from build123d import *

# Parameters (mm, degrees)
PAD_DEPTH    = 4
PAD001_DEPTH = 3
POCKET_DEPTH = 7.001


with BuildPart() as part:
    # Sketch → Pad (new body)
    with BuildSketch(Plane.XY):
        with BuildLine():
            ThreePointArc((0, 3.5), (-3.5, 0), (0, -3.5))
            Line((0, -3.5), (10, -3.5))
            ThreePointArc((10, -3.5), (13.5, 0), (10, 3.5))
            Line((0, 3.5), (10, 3.5))
        make_face()
    extrude(amount=PAD_DEPTH)

    # Sketch001 (on Face6 of Pad) → Pad001 (join)
    with BuildSketch(Plane.XY.offset(4)):
        with BuildLine():
            ThreePointArc((0, 1.85), (-1.85, 0), (0, -1.85))
            Line((0, -1.85), (10, -1.85))
            ThreePointArc((10, -1.85), (11.85, 0), (10, 1.85))
            Line((0, 1.85), (10, 1.85))
        make_face()
    extrude(amount=PAD001_DEPTH)

    # Sketch002 (on Face11 of Pad001) → Pocket (cut, through all)
    with BuildSketch(Plane.XY.offset(7)):
        with BuildLine():
            ThreePointArc((8.35, 0), (6.6, 1.75), (4.85, 0))
            Line((4.85, -3.5), (4.85, 0))
            Line((8.35, -3.5), (4.85, -3.5))
            Line((8.35, 0), (8.35, -3.5))
        make_face()
    extrude(amount=-POCKET_DEPTH, mode=Mode.SUBTRACT)


solid = part.part
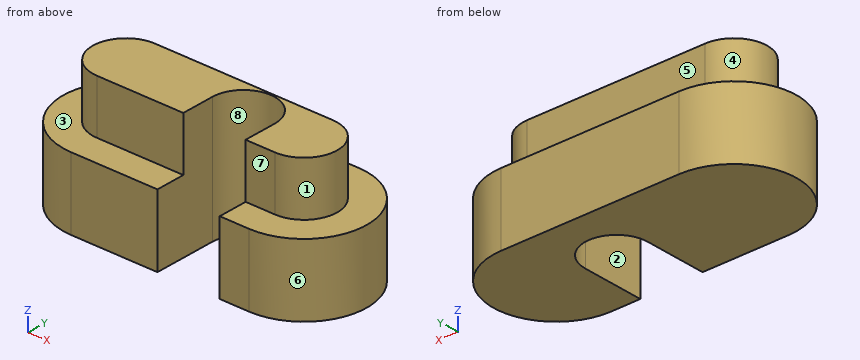
Check sheet for the modelled part. Datum: model origin and axes. Units: mm. Face numbers are marked on the shaded views. A direction names the side the tool comes from. Round coordinates to 2 decimals unless told otherwise and drop trailing zeros. Loops run counter-clockwise (first coordinate to the right, second up) from the corner with the lowest first, then second, coordinate; pieces in that order, holes last. Notation, with made-up numbers: M 30,49.5 L 63,49.5 A9 ccw 63,58.5 Z; hole C -17,37 d1. An arc over 180 degrees is marked long. One line per item, written item: value.
(1) Sectioned sample at A-A, the plane y = -1. Record the cut outline in (x, z), then the cut area to 3 significant figures.
Computed values:
outline: M -3.35,0 L 4.85,0 L 4.85,7 L -1.56,7 L -1.56,4 L -3.35,4 Z; M 8.35,0 L 13.35,0 L 13.35,4 L 11.56,4 L 11.56,7 L 8.35,7 Z
area: 81.7 mm^2
(2) Sectioned sample at D-D, the plane y = -0.25. Record the cut outline in (x, z).
Computed values:
outline: M -3.49,0 L 4.85,0 L 4.85,7 L -1.83,7 L -1.83,4 L -3.49,4 Z; M 8.35,0 L 13.49,0 L 13.49,4 L 11.83,4 L 11.83,7 L 8.35,7 Z
(3) Thickness scan on line 1 (X direction, y = 1.5, z = 5.75); line 2 (X direction, y = -2.75, z = 3.5); line 3 (Z direction, x = 0.25, y = 2.75). Record the ranges inside material, lowest first.
Computed values:
line 1: x = -1.08 to 5.7, 7.5 to 11.08
line 2: x = -2.17 to 4.85, 8.35 to 12.17
line 3: z = 0 to 4
(4) Sectioned sample at B-B, the plane x = 1.25. Record the cut outline in (y, z), then the cut area to 3 significant figures.
Computed values:
outline: M -3.5,0 L 3.5,0 L 3.5,4 L 1.85,4 L 1.85,7 L -1.85,7 L -1.85,4 L -3.5,4 Z
area: 39.1 mm^2
(5) Access from +Z, -Z, +X, -X, +Y, -Y to the whole of each face (thin tool, end or side, straight path). Record for the marked faces 1, 2, 3, 4 and 5.
Computed values:
face 1: +Z, +X
face 2: +Z, -Z, -Y
face 3: +Z
face 4: +Z, -X
face 5: +Z, +X, -X, +Y
(6) Release check for a two-part mould opening along X. For the marked faces 6, 7 and 8 record: +X half, -X half, draft (parallel to the pull), parting line (faces both ways), or undercut.
Computed values:
face 6: +X half
face 7: draft
face 8: undercut
(7) Sectioned sample at C-C, the plane z = 5. Record the cut outline in (x, y).
Computed values:
outline: M 0,-1.85 L 4.85,-1.85 L 4.85,0 A1.75 cw 8.35,0 L 8.35,-1.85 L 10,-1.85 A1.85 ccw 10,1.85 L 0,1.85 A1.85 ccw Z
(8) Depth check by flat-ended pin: pin 1 Ø3 at (y, z) = (-2.5, 2.5) entering from +X; pin 2 Ø1.8 at (y, z) = (-2, 4.5) entering from -X; pin 3 Ø1.5 at (x, z) = (5.5, 6) entering from +Y. Enter the tip coordinate at first touch or a pass-through.
Computed values:
pin 1: stops at x = 13.35
pin 2: stops at x = -3.27
pin 3: stops at y = 1.85
